Can you work these out from the model? Positions are in its coordinate system, mm. Face numbers are marked on the shaded views. A direction names the side the tool comes from. Give positions to 0.01 mm unless a question says otherwise; leave off trailing zeros. Write each loop counter-clockwise with the first axis right and the second up, starting at its lowest first coordinate (ties: lowest second). Pieces come first, ordered by that corner, then holes.
1. Thinking about a two-plate mould opening in Y: for the marked faces 3 and 4, which applies, pulls with the +Y half, pulls with the -Y half, needs draft (parallel to the pull), parting line crosses it, or undercut?
2. On a 3-axis mill with a long thin cutter (end or side, diameter ignored), from which of +Z, -Z, +X, -X, +Y, -Y can I reach the whole of each face in a straight line? I mean the marked faces 1 and 2. Say none if no direction works.
3. I'm going to push flat-ended pins straight in: pin 1 (1 mm diameter, centred on y = -5.5, z = 12.5, fed in from +X); pin 2 (18 mm diameter, centred on x = 0, y = 0, fed in from +Z); pin 3 (5 mm diameter, centred on y = 10.5, z = 3.5, fed in from +X); pin 4 (8 mm diameter, centred on x = -3, z = 14.5, fed in from +Y). Where does each tip first touch, or does it pass through?
4. Suppose I cut it at A-A (x = 0). Please give me the cut outline in (y, z).
5. If I drill on probe 1 along Y at (x, z) = (2.5, 1); probe 2 along Y at (x, z) = (0, 9.75); probe 3 along Y at (x, z) = (0, 2.35), over which ranges is the centre line in solid material (lowest first)?
6. Suppose I cut it at C-C (z = 5). Please give me the cut outline in (x, y), and give its area (3 significant figures).
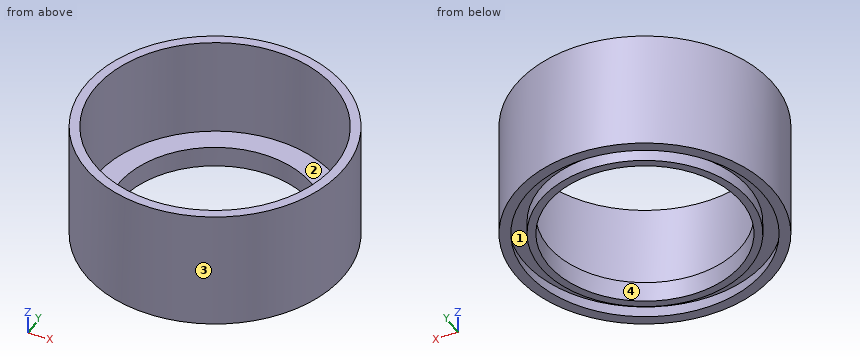
```python
from build123d import *


with BuildPart() as part:
    # Sketch → Revolution (revolve)
    with BuildSketch(Plane.XZ):
        Polygon((16, 0), (16, 2), (18.6, 2), (18.2, 0), (19.8, 0), (19.8, 18.5), (18.35, 18.5), (18.35, 3.2), (14.8, 3.2), (14.8, 0), align=None)
    revolve(axis=Axis((0, 0, 0), (0, 0, 1)))


solid = part.part
```
Checks:
1. face 3: parting line crosses it
1. face 4: undercut
2. face 1: none
2. face 2: +Z
3. pin 1: stops at x = 19.16
3. pin 2: passes through
3. pin 3: stops at x = 18.11
3. pin 4: stops at y = 19.8
4. outline: (-19.8, 0) - (-18.2, 0) - (-18.6, 2) - (-16, 2) - (-16, 0) - (-14.8, 0) - (-14.8, 3.2) - (-18.35, 3.2) - (-18.35, 18.5) - (-19.8, 18.5) - close; (14.8, 0) - (16, 0) - (16, 2) - (18.6, 2) - (18.2, 0) - (19.8, 0) - (19.8, 18.5) - (18.35, 18.5) - (18.35, 3.2) - (14.8, 3.2) - close
5. probe 1: y = -19.64 to -18.23, -15.8 to -14.59, 14.59 to 15.8, 18.23 to 19.64
5. probe 2: y = -19.8 to -18.35, 18.35 to 19.8
5. probe 3: y = -19.8 to -14.8, 14.8 to 19.8
6. outline: circle Ø39.6 at (0, 0); hole circle Ø36.7 at (0, 0)
6. area: 174 mm2
